```python
from build123d import *

# Parameters (mm, degrees)
F0_W     = 88.9
F0_H     = 38.1
F2_DEPTH = 50.8
F1_W     = 63.5
F1_H     = 25.4
F3_DEPTH = 50.801
F4_W     = 44.45
F4_H     = 25.4
F5_DEPTH = 38.101
F6_R     = 6.35
F7_DEPTH = 12.701


with BuildPart() as f2:
    # F0 (on Front) → F2 (new body)
    with BuildSketch(Plane.XZ):
        Rectangle(F0_W, F0_H)
    extrude(amount=F2_DEPTH)

    # F1 (on face) → F3 (cut, through all)
    with BuildSketch(Plane.XZ):
        with Locations((0, 6.35)):
            Rectangle(F1_W, F1_H)
    extrude(amount=F3_DEPTH, mode=Mode.SUBTRACT)

    # F4 (on face) → F5 (cut, through all)
    with BuildSketch(Plane.XY.offset(19.05)):
        with Locations((22.225, -38.1)):
            Rectangle(F4_W, F4_H)
    extrude(amount=-F5_DEPTH, mode=Mode.SUBTRACT)

    # F6 (on face) → F7 (cut, through all)
    with BuildSketch(Plane.XY.offset(-6.35)):
        with Locations((-19.05, -38.1)):
            Circle(F6_R)
        with Locations((6.35, -12.7)):
            Circle(F6_R)
    extrude(amount=-F7_DEPTH, mode=Mode.SUBTRACT)


solid = f2.part
```
The model under review builds one solid part; all positions refer to its coordinate system, in mm. A direction names the side the tool comes from. Give positions to 0.01 mm unless a question says otherwise; leave off trailing zeros. Write each loop counter-clockwise with the first axis right and the second up, starting at its lowest first coordinate (ties: lowest second). Pieces come first, ordered by that corner, then holes.
(1) Consider section B-B, the plane y = -12.7. Give the boundary of the cut face in (x, z), and give its area (3 significant figures).
(2) The part is to be moulded in two halves that separate along Y. For faces 4 (the flat face through (38, -13, 19.05)), 5 (the cylindrical face through (4.97, -18.9, -12.61)), 6 (the cylindrical face through (-25.394, -37.821, -12.611)), 7 (the flat face through (27, -25.4, -8)), say which applies: released by +Y, released by -Y, zero draft, split by the parting line, or undercut.
(3) Consider section A-A, the plane x = 6.35. Give the boundary of the cut face in (y, z).
(4) To check wall thickness, follow L1, parallel to Y at x = -19, z = -13; L2, parallel to Y at x = 6, z = -10; L3, parallel to X at y = -23, z = 16. State the ranges of each line that lie inside material, in increasing order.
(5) Consider section D-D, the plane z = -15. Give the boundary of the cut face in (x, y), and give its area (3 significant figures).
(6) Consider section C-C, the plane z = 0.5. Give the boundary of the cut face in (x, y).
(7) Tool access review of faces 1 (the flat face through (-31.75, -25, 6)), 2 (the flat face through (0, -38, -13)), 3 (the flat face through (-11, -19, -19.05)): name each direction out of +Z, -Z, +X, -X, +Y, -Y from which nothing blocks a thin tool from reaching the whole face with its end or side.
(8) For P1, Ø11.5, axis at x = 29.5, z = -8.5, coming from the -Y side; P2, Ø20.5, axis at x = 6.35, y = -12.7, coming from the -Z side; P3, Ø8, axis at x = -2, y = -14.5, coming from the +Z side; P4, Ø14, axis at y = -39.5, z = -13, coming from the +X side, all flat-tipped, find the tip position at first contact; note any pin that passes through.
Returned:
1. outline: (-44.45, -19.05) - (0, -19.05) - (0, -6.35) - (-31.75, -6.35) - (-31.75, 19.05) - (-44.45, 19.05) - close; (12.7, -19.05) - (44.45, -19.05) - (44.45, 19.05) - (31.75, 19.05) - (31.75, -6.35) - (12.7, -6.35) - close
1. area: 1,610 mm2
2. face 4: zero draft
2. face 5: undercut
2. face 6: undercut
2. face 7: released by -Y
3. outline: (-25.4, -19.05) - (-19.05, -19.05) - (-19.05, -6.35) - (-25.4, -6.35) - close; (-6.35, -19.05) - (0, -19.05) - (0, -6.35) - (-6.35, -6.35) - close
4. L1: y = -50.8 to -44.45, -31.75 to 0
4. L2: y = -25.4 to -19.04, -6.36 to 0
4. L3: x = -44.45 to -31.75, 31.75 to 44.45
5. outline: (-44.45, -50.8) - (0, -50.8) - (0, -25.4) - (44.45, -25.4) - (44.45, 0) - (-44.45, 0) - close; hole circle Ø12.7 at (-19.05, -38.1); hole circle Ø12.7 at (6.35, -12.7)
5. area: 3,130 mm2
6. outline: (-44.45, -50.8) - (-31.75, -50.8) - (-31.75, 0) - (-44.45, 0) - close; (31.75, -25.4) - (44.45, -25.4) - (44.45, 0) - (31.75, 0) - close
7. face 1: +Z, +Y, -Y
7. face 2: +Z, -Z, +X, -Y
7. face 3: -Z, +X, -X, +Y, -Y
8. P1: stops at y = -25.4
8. P2: stops at z = -19.05
8. P3: stops at z = -6.35
8. P4: stops at x = 0
